Autodesk Inventor part; units mm, degrees
ref_plane "YZ Plane" through (0, 0, 0) normal (1, 0, 0) x (0, 1, 0)
ref_plane "XZ Plane" through (0, 0, 0) normal (0, 1, 0) x (-1, 0, 0)
ref_plane "XY Plane" through (0, 0, 0) normal (0, 0, 1) x (1, 0, 0)
sketch "스케치1" plane through (0, 0, 0) normal (0, 0, 1) x (1, 0, 0)
  line L0 (0, 30) -> (120, 30)
  line L1 (120, 30) -> (120, 0)
  line L2 (120, 0) -> (0, 0)
  line L3 (0, 0) -> (0, 30)
  dimension "d0" = 120
  dimension "d1" = 30
extrude "돌출1" add sketch "스케치1" along normal blind 15
sketch "스케치2" plane through (0, 0, 15) normal (0, 0, 1) x (1, 0, 0)
  circle A0 centre (30, 15) radius 7.5
  line L0 (120, 30) -> (0, 30)
  point P0 (0, 0)
  dimension "d4" = 15
  dimension "d5" = 15
sketch "스케치3" plane through (0, 0, 15) normal (0, 0, 1) x (1, 0, 0)
  circle A0 centre (60, 14.5644) radius 7.5
  line L0 (0, 30) -> (0, 0)
  dimension "d8" = 60
extrude "돌출2" cut sketch "스케치3" against normal up to surface (15 mm away)
properties part number "lever1.2"
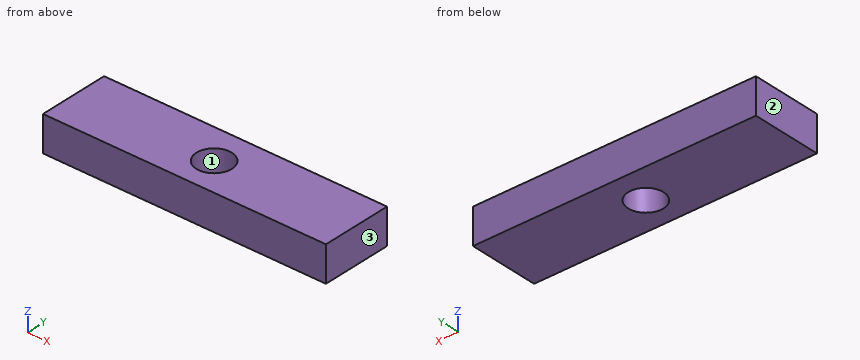
The listing builds one solid part. Answer for the finished solid, in the listing's coordinates (mm). Face numbers are marked on the shaded views. Coordinates: 2 decimals unless noted, no trailing zeros. Write each loop counter-clockwise with the first axis right and the second up, starting at its lowest first coordinate (ties: lowest second). Pieces come first, ordered by that corner, then holes.
Q1. Section B-B, the plane y = 17.75 is taken. Write down the section's boundary in (x, z), then the cut area to 3 significant figures.
Returned:
outline: (0, 0) - (53.21, 0) - (53.21, 15) - (0, 15) - close; (66.79, 0) - (120, 0) - (120, 15) - (66.79, 15) - close
area: 1,600 mm2
Q2. The mould has two halves that part along X. Classify the marked faces 1, 2 and 3: released by +X, released by -X, zero draft, split by the parting line, or undercut.
Returned:
face 1: undercut
face 2: released by -X
face 3: released by +X
Q3. Find the intervals of material crossed by line 1 along Y through (x, z) = (60.5, 6); line 2 along Y through (x, z) = (60, 10.5); line 3 along X through (y, z) = (15, 3.5), in increasing order.
Returned:
line 1: y = 0 to 7.08, 22.05 to 30
line 2: y = 0 to 7.06, 22.06 to 30
line 3: x = 0 to 52.51, 67.49 to 120
Q4. Section A-A, the plane x = 60 is taken. Write down the section's boundary in (y, z), then the cut area to 3 significant figures.
Returned:
outline: (0, 0) - (7.06, 0) - (7.06, 15) - (0, 15) - close; (22.06, 0) - (30, 0) - (30, 15) - (22.06, 15) - close
area: 225 mm2
Q5. Section C-C, the plane z = 1.5 is taken. Write down the section's boundary in (x, y), then the cut area to 3 significant figures.
Returned:
outline: (0, 0) - (120, 0) - (120, 30) - (0, 30) - close; hole circle Ø15 at (60, 14.56)
area: 3,420 mm2
